from build123d import *

# Parameters (mm, degrees)
F0_R     = 18.554146
F1_DEPTH = 20.96888
F2_R     = 35.841286
F3_DEPTH = 53.82837
F5_R     = 22.098703
F6_DEPTH = 20.12846


with BuildPart() as f1:
    # F0 (on Top) → F1 (new body)
    with BuildSketch(Plane.XY):
        Circle(F0_R)
    extrude(amount=F1_DEPTH)

    # F2 (on Top) → F3 (join)
    with BuildSketch(Plane.XY):
        Circle(F2_R)
    extrude(amount=-F3_DEPTH)

    # F5 (on face) → F6 (join)
    with BuildSketch(Plane(origin=(0, 0, -53.82837), x_dir=(1, 0, 0), z_dir=(0, 0, -1))):
        Circle(F5_R)
    extrude(amount=F6_DEPTH)


solid = f1.part
The listing builds one solid part. Answer for the finished solid, in the listing's coordinates (mm). A direction names the side the tool comes from. Round coordinates to 2 decimals unless told otherwise and drop trailing zeros. Order: outer loops, then holes, each group sorted by start corner. A loop starts at its lowest first (then second) coordinate and runs counter-clockwise, first axis right, second up. Notation, with made-up numbers: (39, 62) -> (91, 62) arc R17 cw to (91, 70) -> close; hole circle Ø10 at (-21, 47). An arc over 180 degrees is marked (long way). Write each question's results on one line, items separated by ' | '. Start each with the question number.
Q1. Find section D-D (y = 31.5). Determine the outline of the cut face in (x, z), then the cut area to 3 significant figures.
Q2. Find section A-A (y = 0). Determine the outline of the cut face in (x, z).
Q3. Each of these flat-tipped pins is pushed along its axis until it touches: pin 1 (5 mm diameter, centred on y = 28.5, z = -17.5, fed in from -X); pin 2 (4 mm diameter, centred on y = -11.5, z = -13.5, fed in from +X); pin 3 (4 mm diameter, centred on x = -9.5, z = -63, fed in from -Y). Where does it stop, or does it pass through?
Q4. Which of the six approach directions +Z, -Z, +X, -X, +Y, -Y give full straight-line access (tool end or side, diameter ignored) to faces 1 (the cylindrical face through (34.186, 10.766, -26.537)), 2 (the flat face through (-16.4, -15.4, -53.828)), 3 (the cylindrical face through (-2.4, 18.4, 10.3))?
Q5. Find section C-C (z = -45). Determine the outline of the cut face in (x, y).
Q6. Straight lines are drawn through the part: probe 1 along Z at (x, y) = (-33, -8); probe 2 along Y at (x, z) = (-1, -62); probe 3 along Z at (x, y) = (21, 4). For each, find the intervals that lie inside material, in ascending order. Write a range as from..to.
Worked answers:
1) outline: (-17.1, -53.83) -> (17.1, -53.83) -> (17.1, 0) -> (-17.1, 0) -> close | area: 1,840 mm2
2) outline: (-35.84, -53.83) -> (-22.1, -53.83) -> (-22.1, -73.96) -> (22.1, -73.96) -> (22.1, -53.83) -> (35.84, -53.83) -> (35.84, 0) -> (18.55, 0) -> (18.55, 20.97) -> (-18.55, 20.97) -> (-18.55, 0) -> (-35.84, 0) -> close
3) pin 1: stops at x = -24.67 | pin 2: stops at x = 34.56 | pin 3: stops at y = -20.79
4) face 1: +Z, -Z | face 2: -Z | face 3: +Z
5) outline: circle Ø71.68 at (0, 0)
6) probe 1: z = -53.83..0 | probe 2: y = -22.08..22.08 | probe 3: z = -73.96..0
